The listing builds one solid part. Answer for the finished solid, in the listing's coordinates (mm). Face numbers are marked on the shaded views. A direction names the side the tool comes from. Coordinates: 2 decimals unless noted, no trailing zeros. Order: outer loops, then holes, each group sorted by start corner. A loop starts at its lowest first (then second) coordinate and runs counter-clockwise, first axis right, second up. Notation, with made-up numbers: (-5, 82.5) -> (-1, 82.5) arc R13 cw to (-1, 98.5) -> close; hole circle Ø8 at (25.25, 36.25). An arc over 180 degrees is marked (long way). Write item = value, one per line.
from build123d import *

# Parameters (mm, degrees)
ESQUISSE1_R           = 1
ESQUISSE1_R_2         = 0.5
BOSS_EXTRU_1_DEPTH    = 0.6
BOSS_EXTRU_2_DEPTH    = 0.5
BOSS_EXTRU_4_DEPTH    = 1.5
ESQUISSE3_R           = 1.5
ESQUISSE3_R_2         = 1
ESQUISSE3_R_3         = 0.65
ESQUISSE3_R_4         = 0.5
BOSS_EXTRU_3_DEPTH    = 0.1
CROQUIS1_W            = 0.446175557
CROQUIS1_H            = 1.332309964
CROQUIS1_W_2          = 0.675567057
CROQUIS1_H_2          = 1.353271183
CORTAR_EXTRUIR1_DEPTH = 17


with BuildPart() as part:
    # Esquisse1 → Boss.-Extru.1 (new, symmetric)
    with BuildSketch(Plane.XY):
        with BuildLine():
            Line((-7.5, -4.031128874), (-7.5, -7.5))
            Line((-7.5, -7.5), (7.5, -7.5))
            Line((7.5, -7.5), (7.5, -4.031128874))
            ThreePointArc((7.5, -4.031128874), (9.88121444, 1.027112473), (5.5, 4.5))
            Line((5.5, 4.5), (-5.5, 4.5))
            ThreePointArc((-5.5, 4.5), (-9.88121444, 1.027112473), (-7.5, -4.031128874))
        make_face()
        with Locations((-8, 0)):
            Circle(ESQUISSE1_R, mode=Mode.SUBTRACT)
        with Locations(Location((8, 0, 0), (0, 0, 180))):
            Circle(ESQUISSE1_R, mode=Mode.SUBTRACT)
        with Locations((-6.35, -6.23)):
            Circle(ESQUISSE1_R_2, mode=Mode.SUBTRACT)
        with Locations((-3.81, -6.23)):
            Circle(ESQUISSE1_R_2, mode=Mode.SUBTRACT)
        with Locations((-1.27, -6.23)):
            Circle(ESQUISSE1_R_2, mode=Mode.SUBTRACT)
        with Locations((1.27, -6.23)):
            Circle(ESQUISSE1_R_2, mode=Mode.SUBTRACT)
        with Locations((3.81, -6.23)):
            Circle(ESQUISSE1_R_2, mode=Mode.SUBTRACT)
        with Locations((6.35, -6.23)):
            Circle(ESQUISSE1_R_2, mode=Mode.SUBTRACT)
    extrude(amount=BOSS_EXTRU_1_DEPTH, both=True)

    # Esquisse2 → Boss.-Extru.2 (add)
    with BuildSketch(Plane.XY.offset(0.6)):
        with BuildLine():
            Line((-1.75, 4.25), (1.75, 4.25))
            ThreePointArc((1.75, 4.25), (6, 0), (1.75, -4.25))
            Line((1.75, -4.25), (-1.75, -4.25))
            ThreePointArc((-1.75, -4.25), (-6, 0), (-1.75, 4.25))
        make_face()
    extrude(amount=BOSS_EXTRU_2_DEPTH)

    # Esquisse4 → Boss.-Extru.4 (add)
    with BuildSketch(Plane.XY.offset(1.1)):
        with BuildLine():
            Line((-1.75, -3.25), (1.75, -3.25))
            ThreePointArc((1.75, -3.25), (5, 0), (1.75, 3.25))
            Line((1.75, 3.25), (-1.75, 3.25))
            ThreePointArc((-1.75, 3.25), (-5, 0), (-1.75, -3.25))
        make_face()
    extrude(amount=BOSS_EXTRU_4_DEPTH)

    # Esquisse3 → Boss.-Extru.3 (add)
    # profile 1 of 8: a face of its own
    with BuildSketch(Plane.XY.offset(0.6)):
        with Locations((-8, 0)):
            Circle(ESQUISSE3_R)
        with Locations((-8, 0)):
            Circle(ESQUISSE3_R_2, mode=Mode.SUBTRACT)
    # profile 2 of 8: a face of its own
    with BuildSketch(Plane.XY.offset(0.6)):
        with Locations((8, 0)):
            Circle(ESQUISSE3_R)
        with Locations(Location((8, 0, 0), (0, 0, 180))):
            Circle(ESQUISSE3_R_2, mode=Mode.SUBTRACT)
    # profile 3 of 8: a face of its own
    with BuildSketch(Plane.XY.offset(0.6)):
        with Locations((-6.35, -6.23)):
            Circle(ESQUISSE3_R_3)
        with Locations((-6.35, -6.23)):
            Circle(ESQUISSE3_R_4, mode=Mode.SUBTRACT)
    # profile 4 of 8: a face of its own
    with BuildSketch(Plane.XY.offset(0.6)):
        with Locations((-3.81, -6.23)):
            Circle(ESQUISSE3_R_3)
        with Locations((-3.81, -6.23)):
            Circle(ESQUISSE3_R_4, mode=Mode.SUBTRACT)
    # profile 5 of 8: a face of its own
    with BuildSketch(Plane.XY.offset(0.6)):
        with Locations((-1.27, -6.23)):
            Circle(ESQUISSE3_R_3)
        with Locations((-1.27, -6.23)):
            Circle(ESQUISSE3_R_4, mode=Mode.SUBTRACT)
    # profile 6 of 8: a face of its own
    with BuildSketch(Plane.XY.offset(0.6)):
        with Locations((1.27, -6.23)):
            Circle(ESQUISSE3_R_3)
        with Locations((1.27, -6.23)):
            Circle(ESQUISSE3_R_4, mode=Mode.SUBTRACT)
    # profile 7 of 8: a face of its own
    with BuildSketch(Plane.XY.offset(0.6)):
        with Locations((3.81, -6.23)):
            Circle(ESQUISSE3_R_3)
        with Locations((3.81, -6.23)):
            Circle(ESQUISSE3_R_4, mode=Mode.SUBTRACT)
    # profile 8 of 8: a face of its own
    with BuildSketch(Plane.XY.offset(0.6)):
        with Locations((6.35, -6.23)):
            Circle(ESQUISSE3_R_3)
        with Locations((6.35, -6.23)):
            Circle(ESQUISSE3_R_4, mode=Mode.SUBTRACT)
    boss_extru_3 = extrude(amount=BOSS_EXTRU_3_DEPTH)

    # Symétrie1: Boss.-Extru.3 across plane
    add(boss_extru_3.mirror(Plane.XY))

    # Croquis1 → Cortar-Extruir1 (cut)
    with BuildSketch(Plane(origin=(7.5, 0, 0), x_dir=(0, 0, -1), z_dir=(1, 0, 0))):
        with Locations((0.823087779, -6.23167244)):
            Rectangle(CROQUIS1_W, CROQUIS1_H)
        with Locations((-0.937783529, -6.256635592)):
            Rectangle(CROQUIS1_W_2, CROQUIS1_H_2)
    extrude(amount=-CORTAR_EXTRUIR1_DEPTH, mode=Mode.SUBTRACT)


solid = part.part
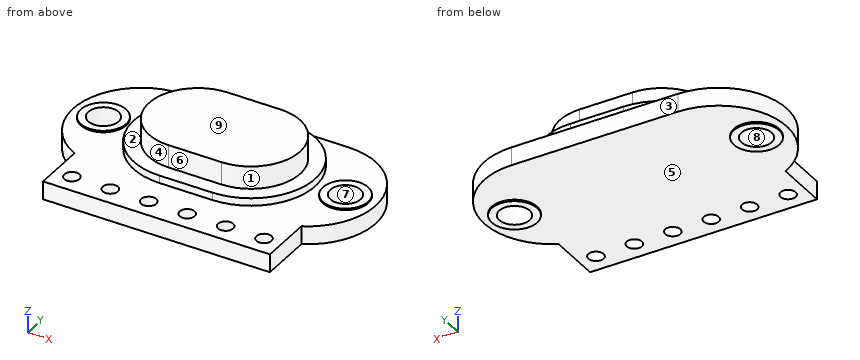
Q1. Section B-B, the plane x = -1.27 is taken. Give the vertices of the cut face in (y, z).
The answers:
outline = (-7.5, -0.6) -> (-6.73, -0.6) -> (-6.73, 0.6) -> (-7.5, 0.6) -> close; (-5.73, -0.6) -> (4.5, -0.6) -> (4.5, 0.6) -> (4.25, 0.6) -> (4.25, 1.1) -> (3.25, 1.1) -> (3.25, 2.6) -> (-3.25, 2.6) -> (-3.25, 1.1) -> (-4.25, 1.1) -> (-4.25, 0.6) -> (-5.73, 0.6) -> close
Q2. Each of these flat-tipped pins is pushed along its axis until it touches: pin 1 Ø2.5 at (x, y) = (-7.5, 0.5) entering from +Z; pin 2 Ø6 at (x, y) = (-2, 0) entering from -Z; pin 3 Ø1 at (y, z) = (-6.5, 0.5) entering from -X. Where does it stop, or does it pass through?
The answers:
pin_1 = 0.7
pin_2 = -0.6
pin_3 = -7.5
Q3. The mould has two halves that part along Y. Classify the marked faces 6, 7, 8 and 9: released by +Y, released by -Y, zero draft, split by the parting line, or undercut.
The answers:
face_6 = released by -Y
face_7 = undercut
face_8 = undercut
face_9 = zero draft
Q4. Find the intervals of material crossed by line 1 along Y through (x, z) = (-1.27, -0.05); line 2 along Z through (x, y) = (-1.5, -5.75); line 3 along Z through (x, y) = (-2.25, -1), in increasing order.
The answers:
line_1 = -7.5 to -6.73, -5.73 to 4.5
line_2 = -0.6 to 0.6
line_3 = -0.6 to 2.6
Q5. Section C-C, the plane y = -1.75 is taken. Give the vertices of the cut face in (x, z), plus the area to 3 significant figures.
The answers:
outline = (-9.65, -0.6) -> (9.65, -0.6) -> (9.65, 0.6) -> (5.62, 0.6) -> (5.62, 1.1) -> (4.49, 1.1) -> (4.49, 2.6) -> (-4.49, 2.6) -> (-4.49, 1.1) -> (-5.62, 1.1) -> (-5.62, 0.6) -> (-9.65, 0.6) -> close
area = 42.2 mm2
Q6. A tool of negligible diameter and unlimited length cuts with its end or side. For the marked faces 1, 2, 3, 4 and 5, from which of +Z, -Z, +X, -X, +Y, -Y can it reach the whole face along a straight path? Write none if from no direction.
The answers:
face_1 = +Z, +X
face_2 = +Z
face_3 = +Z, -Z, +X, -X, +Y
face_4 = +Z, -X
face_5 = -Z
Q7. Section A-A, the plane y = -6.23 is taken. Give the vertices of the cut face in (x, z), plus the area to 3 significant figures.
The answers:
outline = (-7.5, -0.6) -> (-6.85, -0.6) -> (-6.85, 0.6) -> (-7.5, 0.6) -> close; (-5.85, -0.6) -> (-4.31, -0.6) -> (-4.31, 0.6) -> (-5.85, 0.6) -> close; (-3.31, -0.6) -> (-1.77, -0.6) -> (-1.77, 0.6) -> (-3.31, 0.6) -> close; (-0.77, -0.6) -> (0.77, -0.6) -> (0.77, 0.6) -> (-0.77, 0.6) -> close; (1.77, -0.6) -> (3.31, -0.6) -> (3.31, 0.6) -> (1.77, 0.6) -> close; (4.31, -0.6) -> (5.85, -0.6) -> (5.85, 0.6) -> (4.31, 0.6) -> close; (6.85, -0.6) -> (7.5, -0.6) -> (7.5, 0.6) -> (6.85, 0.6) -> close
area = 10.8 mm2
Q8. Section D-D, the plane x = 8.5 is taken. Give the vertices of the cut face in (y, z).
The answers:
outline = (-3.35, -0.6) -> (-1.41, -0.6) -> (-1.41, -0.7) -> (-0.87, -0.7) -> (-0.87, 0.7) -> (-1.41, 0.7) -> (-1.41, 0.6) -> (-3.35, 0.6) -> close; (0.87, -0.7) -> (1.41, -0.7) -> (1.41, -0.6) -> (3.35, -0.6) -> (3.35, 0.6) -> (1.41, 0.6) -> (1.41, 0.7) -> (0.87, 0.7) -> close
